Can you work these out from the model? Positions are in its coordinate system, mm. A direction names the side the tool comes from. Round coordinates to 2 decimals unless told otherwise and drop trailing zeros. Write each loop counter-clockwise with the first axis right and the second up, starting at its lowest first coordinate (ties: lowest second). Pieces come first, ordered by that corner, then holes. Notation, with made-up numbers: M 9,-3 L 15,-3 A21 ccw 15,31 Z; hole C -22.75,61.25 d10. An arc over 180 degrees is marked long. Answer as a JSON object with one key per item and string values. Group by question number.
1) On a 3-axis mill with a long thin cutter (end or side, diameter ignored), from which of +Z, -Z, +X, -X, +Y, -Y can I reach the whole of each face in a straight line? I mean faces 1 (the flat face through (13, 705, -8)), 2 (the cylindrical face through (-4.769, 21.477, 109.3)), 3 (the cylindrical face through (-4.769, 610.56, 21.477)), 4 (the cylindrical face through (-28, 652, 21)). Say none if no direction works.
2) I'm going to push flat-ended pins straight in: pin 1 Ø1.5 at (x, y) = (-22.5, 501) entering from -Z; pin 2 Ø9 at (x, z) = (0, 0.5) entering from +Y; pin 3 Ø1 at (x, y) = (-22.5, 466) entering from -Z. Where does each tip first touch, or does it pass through?
3) Please list where these lines run through material, in increasing order: L1, parallel to X at y = 683.5, z = 0; L2, parallel to Z at x = 0, y = 211; L3, parallel to Y at x = -2, z = 125. Write a range as [from, to].
4) Suppose I cut it at B-B, the plane z = 0. State how many separate pieces and enclosed holes the cut face has, and give its area (3 significant figures).
5) Suppose I cut it at A-A, the plane y = 431. Write out the boundary of the cut face in (x, z).
6) If we mould it in two halves opening along Z, with no side actions, what happens to faces 5 (the cylindrical face through (-13.887, 679.65, 10.648)), 6 (the cylindrical face through (-14.985, 679.65, -0.66)), 7 (the flat face through (-1.7, -22.1, 160)), 8 (the flat face through (-24, 650, -8))? For each: +Z half, -Z half, draft (parallel to the pull), parting line (faces both ways), or undercut.
from build123d import *

# Parameters (mm, degrees)
SKETCH9_R           = 25
SKETCH9_R_2         = 22
SKETCH10_R          = 35
BOSS_EXTRUDE1_DEPTH = 5
SKETCH11_R          = 17.5
SKETCH11_R_2        = 15
EXTRUDE_THIN1_DEPTH = 50


with BuildPart() as part:
    # Sweep-Thin1: sweep along a path in Sketch2
    with BuildLine(Plane(origin=(0, 0, 0), x_dir=(0, 0, -1), z_dir=(1, 0, 0))) as sweep_thin1_path:
        Line((-160, 0), (-60, 0))
        ThreePointArc((-60, 0), (-17.573593129, 17.573593129), (0, 60))
        Line((0, 60), (0, 650))
    # Sketch9 → Sweep-Thin1 (sweep)
    with BuildSketch(Plane(origin=(0, 650, 0), x_dir=(1, 0, 0), z_dir=(0, 1, 0))):
        Circle(SKETCH9_R)
        Circle(SKETCH9_R_2, mode=Mode.SUBTRACT)
    sweep(path=sweep_thin1_path.line)

    # Sketch10 → Boss-Extrude1 (add)
    with BuildSketch(Plane(origin=(0, 650, 0), x_dir=(1, 0, 0), z_dir=(0, 1, 0))):
        Circle(SKETCH10_R)
    boss_extrude1 = extrude(amount=BOSS_EXTRUDE1_DEPTH)

    # Sketch11 → Extrude-Thin1 (add)
    with BuildSketch(Plane(origin=(0, 655, 0), x_dir=(1, 0, 0), z_dir=(0, 1, 0))):
        Circle(SKETCH11_R)
        Circle(SKETCH11_R_2, mode=Mode.SUBTRACT)
    extrude(amount=EXTRUDE_THIN1_DEPTH)

    # Mirror1: Boss-Extrude1 across plane
    add(boss_extrude1.mirror(Plane.ZX.offset(610)))


solid = part.part
Results:
{
 "1": {"face 1": "+Z, -Z, +X, -X, +Y", "face 2": "+Z", "face 3": "none", "face 4": "+Y"},
 "2": {"pin 1": "z = -12.33", "pin 2": "y = 655", "pin 3": "z = -11.87"},
 "3": {"L1": "[-17.5, -15], [15, 17.5]", "L2": "[-25, -22], [22, 25]", "L3": "[-24.92, -21.91], [21.91, 24.92]"},
 "4": {"separate pieces": "1", "enclosed holes": "2", "area": "4,930 mm^2"},
 "5": {"outline": "C 0,0 d50; hole C 0,0 d44"},
 "6": {"face 5": "parting line", "face 6": "undercut", "face 7": "+Z half", "face 8": "draft"}
}
